The listing builds one solid part. Answer for the finished solid, in the listing's coordinates (mm). Face numbers are marked on the shaded views. A direction names the side the tool comes from. Coordinates: 2 decimals unless noted, no trailing zeros. Order: outer loops, then holes, each group sorted by start corner. A loop starts at its lowest first (then second) coordinate and runs counter-clockwise, first axis right, second up.
```python
from build123d import *

# Parameters (mm, degrees)
SKETCH2_W            = 42
SKETCH2_H            = 37
BOSS_EXTRUDE1_DEPTH  = 19
FILLET1_R            = 1
FILLET2_R            = 1
SKETCH3_W            = 2.2
SKETCH3_H            = 8.5
BOSS_EXTRUDE2_DEPTH  = 6
SKETCH4_W            = 6
SKETCH4_H            = 1
BOSS_EXTRUDE3_DEPTH  = 1
CHAMFER1_SIZE2       = 1
CHAMFER1_SIZE        = 6
FILLET3_R            = 1
CUT_EXTRUDE1_DEPTH   = 6
FILLET3_OF_MIRROR9_R = 1
CHAMFER2_SIZE        = 1
CHAMFER2_SIZE_2      = 6
FILLET4_R            = 1
BOSS_EXTRUDE4_DEPTH  = 2
SKETCH9_R            = 6.574433214
BOSS_EXTRUDE5_DEPTH  = 1
SKETCH10_R           = 5.689687475
BOSS_EXTRUDE6_DEPTH  = 0.7
SKETCH11_R           = 1.55
CUT_EXTRUDE2_DEPTH   = 10


# Some blends are built 0.0001 mm under size
with BuildPart() as part:
    # Sketch2 → Boss-Extrude1 (new body)
    with BuildSketch(Plane(origin=(0, 0, 0), x_dir=(1, 0, 0), z_dir=(0, 1, 0))):
        with Locations((-10.021609405, 3.404712932)):
            Rectangle(SKETCH2_W, SKETCH2_H)
    extrude(amount=BOSS_EXTRUDE1_DEPTH)

    # Fillet1
    fillet1_edges = [part.edges().sort_by_distance(p)[0] for p in [
        (10.978390595, 19, -3.404712932),
    ]]
    fillet(fillet1_edges, radius=FILLET1_R)

    # Fillet2
    fillet2_edges = [part.edges().sort_by_distance(p)[0] for p in [
        (-31.021609405, 19, -3.404712932),
        (10.978390595, 0, -3.404712932),
        (-31.021609405, 0, -3.404712932),
    ]]
    fillet(fillet2_edges, radius=FILLET2_R)

    # Sketch3 → Boss-Extrude2 (add)
    with BuildSketch(Plane(origin=(10.978390595, 0, 0), x_dir=(0, 0, -1), z_dir=(1, 0, 0))):
        with Locations((15.004712932, 5.25)):
            Rectangle(SKETCH3_W, SKETCH3_H)
        with Locations((15.004712932, 13.75)):
            Rectangle(SKETCH3_W, SKETCH3_H)
    boss_extrude2 = extrude(amount=BOSS_EXTRUDE2_DEPTH)

    # Sketch4 → Boss-Extrude3 (add)
    with BuildSketch(Plane(origin=(0, 0, -16.104712932), x_dir=(-1, 0, 0), z_dir=(0, 0, -1))):
        with Locations((-13.978390595, 9.5)):
            Rectangle(SKETCH4_W, SKETCH4_H)
    boss_extrude3 = extrude(amount=BOSS_EXTRUDE3_DEPTH)

    # Chamfer1
    chamfer1_edges = [part.edges().sort_by_distance(p)[0] for p in [
        (16.978390595, 9.5, -17.104712932),
    ]]
    chamfer1_side = [part.faces().sort_by_distance(p)[0] for p in [
        (16.958390595, 9.5, -17.104712932),
    ]]
    chamfer(chamfer1_edges, length=CHAMFER1_SIZE - 0.0001, length2=CHAMFER1_SIZE2 - 0.0001, reference=chamfer1_side[0])  # a hair under: the kernel refuses the full size

    # Fillet3
    fillet3_edges = [part.edges().sort_by_distance(p)[0] for p in [
        (16.978390595, 18, -15.004712932),
        (16.978390595, 1, -15.004712932),
    ]]
    fillet(fillet3_edges, radius=FILLET3_R)

    # Sketch5 → Cut-Extrude1 (cut)
    with BuildSketch(Plane(origin=(0, 0, -16.104712932), x_dir=(-1, 0, 0), z_dir=(0, 0, -1))):
        with BuildLine():
            Line((-16.978390595, 15.5), (-16.978390595, 13.5))
            Line((-16.978390595, 13.5), (-16.710441403, 13.5))
            ThreePointArc((-16.710441403, 13.5), (-12.978390595, 14.5), (-16.710441403, 15.5))
            Line((-16.710441403, 15.5), (-16.978390595, 15.5))
        make_face()
        with BuildLine():
            Line((-16.978390595, 3.5), (-16.978390595, 5.5))
            Line((-16.978390595, 5.5), (-16.710441403, 5.5))
            ThreePointArc((-16.710441403, 5.5), (-12.978390595, 4.5), (-16.710441403, 3.5))
            Line((-16.710441403, 3.5), (-16.978390595, 3.5))
        make_face()
    cut_extrude1 = extrude(amount=-CUT_EXTRUDE1_DEPTH, mode=Mode.SUBTRACT)

    # Mirror9: Boss-Extrude2, Boss-Extrude3, Cut-Extrude1 across plane
    add(boss_extrude2.mirror(Plane(origin=(-10.021609405, 0, 0), x_dir=(0, 0, 1), z_dir=(1, 0, 0))))
    add(boss_extrude3.mirror(Plane(origin=(-10.021609405, 0, 0), x_dir=(0, 0, 1), z_dir=(1, 0, 0))))
    add(cut_extrude1.mirror(Plane(origin=(-10.021609405, 0, 0), x_dir=(0, 0, 1), z_dir=(1, 0, 0))), mode=Mode.SUBTRACT)

    # Fillet3 of Mirror9
    fillet3_of_mirror9_edges = [part.edges().sort_by_distance(p)[0] for p in [
        (-37.021609405, 18, -15.004712932),
        (-37.021609405, 1, -15.004712932),
    ]]
    fillet(fillet3_of_mirror9_edges, radius=FILLET3_OF_MIRROR9_R)

    # Chamfer2
    # the kernel refuses this chamfer: 6, 1 mm, written as the material it takes off along each edge
    with BuildSketch(Plane(origin=(-37.021609405, 25.592148365, -17.104712932), x_dir=(-0.22206223681747272, 0, 0.9750324932942598), z_dir=(0, -1, 0))) as chamfer2_piece_1:
        Polygon((CHAMFER2_SIZE * 0.975032493294, -CHAMFER2_SIZE * 0.222062236817), (-CHAMFER2_SIZE_2 * 0.222062236817, -CHAMFER2_SIZE_2 * 0.975032493294), (0, 0), align=None)
    extrude(amount=32.18429673, mode=Mode.SUBTRACT)

    # Fillet4
    fillet4_edges = [part.edges().sort_by_distance(p)[0] for p in [
        (10.978390595, 9.5, 15.095287068),
        (10.685497376, 18.707106781, 15.095287068),
        (-10.021609405, 19, 15.095287068),
        (-31.021609405, 9.5, 15.095287068),
        (-10.021609405, 0, 15.095287068),
        (10.685497376, 0.292893219, 15.095287068),
        (-30.728716186, 0.292893219, 15.095287068),
        (-30.728716186, 18.707106781, 15.095287068),
    ]]
    fillet(fillet4_edges, radius=FILLET4_R)

    # Sketch8 → Boss-Extrude4 (add)
    with BuildSketch(Plane(origin=(0, 0, -21.904712932), x_dir=(-1, 0, 0), z_dir=(0, 0, -1))):
        with BuildLine():
            Line((2.924068209, 18.707106781), (23.752988448, 18.707106781))
            Line((23.752988448, 18.707106781), (23.752988448, 14.023415458))
            ThreePointArc((23.752988448, 14.023415458), (25.81960193, 9.5), (23.752988448, 4.976584542))
            Line((23.752988448, 4.976584542), (23.752988448, 0.292893219))
            Line((23.752988448, 0.292893219), (2.924068209, 0.292893219))
            ThreePointArc((2.924068209, 0.292893219), (-10.978390595, 9.5), (2.924068209, 18.707106781))
        make_face()
    extrude(amount=BOSS_EXTRUDE4_DEPTH)

    # Sketch9 → Boss-Extrude5 (add)
    with BuildSketch(Plane(origin=(0, 0, -23.904712932), x_dir=(-1, 0, 0), z_dir=(0, 0, -1))):
        with Locations((-0.978390595, 9.5)):
            Circle(SKETCH9_R)
    extrude(amount=BOSS_EXTRUDE5_DEPTH)

    # Sketch10 → Boss-Extrude6 (add)
    with BuildSketch(Plane(origin=(0, 0, -24.904712932), x_dir=(-1, 0, 0), z_dir=(0, 0, -1))):
        with Locations((-0.978390595, 9.5)):
            Circle(SKETCH10_R)
    extrude(amount=BOSS_EXTRUDE6_DEPTH)

    # Sketch11 → Cut-Extrude2 (cut)
    with BuildSketch(Plane(origin=(0, 0, -25.604712932), x_dir=(-1, 0, 0), z_dir=(0, 0, -1))):
        with Locations((-0.978390595, 9.5)):
            Circle(SKETCH11_R)
    extrude(amount=-CUT_EXTRUDE2_DEPTH, mode=Mode.SUBTRACT)


solid = part.part
```
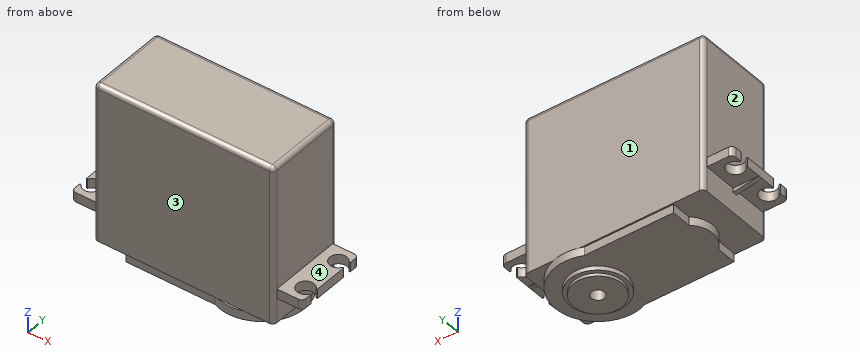
(1) Each of these flat-tipped pins is pushed along its axis until it touches: pin 1 Ø11 at (x, z) = (-17.5, 2) entering from +Y; pin 2 Ø6 at (x, z) = (-25, -4.5) entering from -Y; pin 3 Ø5 at (x, y) = (-35.02, 4.5) entering from +Z. Where does it stop, or does it pass through?
(2) For the marked faces 1, 2, 3 and 4, determine the directions among +Z, -Z, +X, -X, +Y, -Y from which every point of the face is accessible in a straight line to the end or side of a thin tool.
(3) Find section A-A (z = -21). Write down the section's boundary in (x, y), and give its area (3 significant figures).
(4) Find section B-B (x = -17.5). Write down the section's boundary in (y, z), and give its area (3 significant figures).
(5) Find section C-C (z = -5). Write down the section's boundary in (x, y).
(6) Consider line 1 (X direction, y = 6.25, z = -15); line 2 (Y direction, x = -21, z = -22); line 3 (X direction, y = 6.5, z = -9). Determine where each line is inside the solid, lowest interval first.
(7) Find section D-D (x = -27). Write down the section's boundary in (y, z).
Findings below:
1. pin 1: stops at y = 19
1. pin 2: stops at y = 0
1. pin 3: stops at z = -13.9
2. face 1: +Z, +X, -X, +Y
2. face 2: +Z, -X, +Y, -Y
2. face 3: +Z, +X, -X, -Y
2. face 4: +Z, +X, +Y, -Y
3. outline: (-31.02, 1) arc R1 ccw to (-30.02, 0) - (9.98, 0) arc R1 ccw to (10.98, 1) - (10.98, 18) arc R1 ccw to (9.98, 19) - (-30.02, 19) arc R1 ccw to (-31.02, 18) - close; hole circle Ø3.1 at (0.98, 9.5)
3. area: 790 mm2
4. outline: (0, -21.9) - (0.29, -21.9) - (0.29, -23.9) - (18.71, -23.9) - (18.71, -21.9) - (19, -21.9) - (19, 14.1) arc R1 ccw to (18, 15.1) - (1, 15.1) arc R1 ccw to (0, 14.1) - close
4. area: 739 mm2
5. outline: (-31.02, 1) arc R1 ccw to (-30.02, 0) - (9.98, 0) arc R1 ccw to (10.98, 1) - (10.98, 18) arc R1 ccw to (9.98, 19) - (-30.02, 19) arc R1 ccw to (-31.02, 18) - close
6. line 1: x = -37.02 to -35.99, -34.05 to 14.01, 15.95 to 16.98
6. line 2: y = 0.29 to 18.71
6. line 3: x = -31.02 to 10.98
7. outline: (0, -21.9) - (19, -21.9) - (19, 14.1) arc R1 ccw to (18, 15.1) - (1, 15.1) arc R1 ccw to (0, 14.1) - close
